Model file for the job. Use its own axes, mm. A direction names the side the tool comes from. Give positions to 0.01 mm unless a question says otherwise; leave off trailing zeros. Write each loop counter-clockwise with the first axis right and the second up, starting at its lowest first coordinate (ties: lowest second). Pieces come first, ordered by that corner, then holes. Notation, with made-up numbers: (-10.75, 53) - (36.25, 53) arc R10 ccw to (36.25, 62) - close; hole circle Ø9 at (72, 59). An arc over 180 degrees is marked (long way). Use a Markdown table: item, result. Add a question column.
```python
from build123d import *

# Parameters (mm, degrees)
PAD_DEPTH    = 20
SKETCH001_R  = 2.2
PAD001_DEPTH = 1
PAD002_DEPTH = 20


with BuildPart() as part:
    # Sketch → Pad (new body)
    with BuildSketch(Plane.XZ):
        with BuildLine():
            Line((-7.5, 7.000023), (-7.5, 0))
            Line((-7.5, 0), (7.5, 0))
            Line((7.5, 0), (7.5, 7.000023))
            ThreePointArc((7.5, 7.000023), (6.929092, 9.870136), (5.303301, 12.303301))
            Line((4.242641, 11.242641), (5.303301, 12.303301))
            ThreePointArc((-4.242641, 11.242641), (0, 1), (4.242641, 11.242641))
            Line((-4.242641, 11.242641), (-5.303301, 12.303301))
            ThreePointArc((-5.303301, 12.303301), (-6.929092, 9.870137), (-7.5, 7.000023))
        make_face()
    extrude(amount=PAD_DEPTH)

    # Sketch001 → Pad001 (new body)
    with BuildSketch(Plane(origin=(0, 0, 0), x_dir=(1, 0, 0), z_dir=(0, 0, -1))):
        with BuildLine():
            ThreePointArc((13.543105, 59.357983), (8, 59.6), (2.456895, 59.357983))
            ThreePointArc((2.456895, 59.357983), (0.439153, 58.514691), (-0.718231, 56.65919))
            Line((-7.5, 20), (-0.718231, 56.65919))
            Line((-7.5, 0), (-7.5, 20))
            Line((6.06439, -7.500488), (-7.5, 0))
            ThreePointArc((6.06439, -7.500488), (9.891476, -7.524531), (11.987014, -4.32205))
            Line((11.987014, -4.32205), (16.817658, 55.481839))
            ThreePointArc((16.817658, 55.481839), (15.979375, 58.094898), (13.543105, 59.357983))
        make_face()
        with Locations((8, -4)):
            Circle(SKETCH001_R, mode=Mode.SUBTRACT)
        with BuildLine():
            ThreePointArc((13.046318, 53.679673), (8, 53.9), (2.953682, 53.679673))
            ThreePointArc((2.587628, 57.863691), (0.678647, 55.588655), (2.953682, 53.679673))
            ThreePointArc((13.412372, 57.863691), (8, 58.1), (2.587628, 57.863691))
            ThreePointArc((13.046318, 53.679673), (15.321353, 55.588655), (13.412372, 57.863691))
        make_face(mode=Mode.SUBTRACT)
    extrude(amount=-PAD001_DEPTH)

    # Sketch002 → Pad002 (new body)
    with BuildSketch(Plane.XZ.offset(20)):
        with BuildLine():
            ThreePointArc((-3.252691, 10.252691), (0, 2.4), (3.252691, 10.252691))
            Line((3.252691, 10.252691), (4.242641, 11.242641))
            ThreePointArc((-4.242641, 11.242641), (0, 1), (4.242641, 11.242641))
            Line((-3.252691, 10.252691), (-4.242641, 11.242641))
        make_face()
    extrude(amount=-PAD002_DEPTH)


solid = part.part
```
(1) Flat gauge pins, fed straight in: pin 1 (3 mm diameter, centred on y = -5, z = 5.5, fed in from +X); pin 2 (6 mm diameter, centred on x = 3.5, z = 6, fed in from +Y); pin 3 (2 mm diameter, centred on x = 11.5, y = -30.5, fed in from +Z). Where does each tip first touch, or does it go through?
(2) Which spindle directions (+Z, -Z, +X, -X, +Y, -Y) get a long thin tool onto all of the face, cutting with end or side? Do faces 5 (the flat face through (-4.157, -38.073, 0.493)), 6 (the cylindrical face through (0.675, -55.635, 0.493)), 7 (the flat face through (0, 0, 2)). Say none if no direction does.
(3) Band-saw the part on D-D (y = -2). Write the cut outline in (x, z).
(4) Two-plate mould, pull along X, no slides. Class faces 1 (the flat face through (-4, -10, 11)), 2 (the flat face through (7.5, -10, 4)), 3 (the flat face through (4, -10, 11)), 4 (the cylindrical face through (-6.913, -9.86, 9.908)): +X half, -X half, draft (parallel to the pull), parting line (faces both ways), or undercut.
(5) Probe probe 1 along Y at (x, z) = (8, 0.7); probe 2 along X at (y, z) = (-9, 7); probe 3 along Y at (x, z) = (-5, 1.25). List the from-to ranges inside material, lowest first. Write a range as [from, to].
(6) Band-saw the part on C-C (x = 0). Write the cut outline in (y, z), then the cut area to 3 significant figures.
(7) Band-saw the part on A-A (z = 8.25). Write the cut outline in (x, y).
(8) Band-saw the part on B-B (y = -11). Write the cut outline in (x, z), then the cut area to 3 significant figures.
Model answer:
| question | item | result |
|---|---|---|
| 1 | pin 1 | stops at x = 7.5 |
| 1 | pin 2 | stops at y = 0 |
| 1 | pin 3 | stops at z = 1 |
| 2 | face 5 | +Z, -Z, -X, -Y |
| 2 | face 6 | +Z, -Z |
| 2 | face 7 | +Z, +X, -X, +Y |
| 3 | outline | (-7.5, 0) - (12.5, 0) - (12.5, 1) - (7.5, 1) - (7.5, 7) arc R7.5 ccw to (5.3, 12.3) - (3.25, 10.25) arc R4.6 cw (long way) to (-3.25, 10.25) - (-5.3, 12.3) arc R7.5 ccw to (-7.5, 7) - close |
| 4 | face 1 | undercut |
| 4 | face 2 | +X half |
| 4 | face 3 | undercut |
| 4 | face 4 | -X half |
| 5 | probe 1 | y = [-59.6, -58.1], [-53.9, 1.8], [6.2, 8] |
| 5 | probe 2 | x = [-7.5, -4.6], [4.6, 7.5] |
| 5 | probe 3 | y = [-20, 0] |
| 6 | outline | (-58.07, 0) - (4.15, 0) - (4.15, 1) - (0, 1) - (0, 2.4) - (-20, 2.4) - (-20, 1) - (-58.07, 1) - close |
| 6 | area | 90.2 mm^2 |
| 7 | outline | (-7.4, -20) - (-4.43, -20) - (-4.43, 0) - (-7.4, 0) - close; (4.43, -20) - (7.4, -20) - (7.4, 0) - (4.43, 0) - close |
| 8 | outline | (-7.5, 0) - (13.22, 0) - (13.22, 1) - (7.5, 1) - (7.5, 7) arc R7.5 ccw to (5.3, 12.3) - (3.25, 10.25) arc R4.6 cw (long way) to (-3.25, 10.25) - (-5.3, 12.3) arc R7.5 ccw to (-7.5, 7) - close |
| 8 | area | 105 mm^2 |
